Answer from the drawing. Dimensions are ordinates in mm from the lowest x, y and z of the part. A direction names the side the tool comes from. Round coordinates to 2 decimals unless told otherwise and drop trailing zeros. Order: outer loops, then holes, each group sorted by start corner. A loop starts at its lowest first (then second) coordinate and runs counter-clockwise, first axis right, second up. Notation, with made-up numbers: (-6, -23) -> (43, -23) arc R15 cw to (43, -13) -> close; hole circle Ø5 at (-26, -16.5). An arc over 180 degrees is marked (long way). Use a Markdown table: item, result. Add a question column.
Item 1: A cutting plane is placed at B-B, the plane y = 14.5. Determine the outline of the cut face in (x, z).
Item 2: A cutting plane is placed at C-C, the plane y = 5.25. Determine the outline of the cut face in (x, z).
Item 3: Flat-ended cylindrical pins translate along their axes: P1, Ø5, axis at x = 4, z = 2, coming from the +Y side; P2, Ø5, axis at x = 17.5, y = 12, coming from the +Z side; P3, Ø5, axis at x = 8, y = 10, coming from the +Z side; P4, Ø6, axis at y = 15, z = 9.5, coming from the +X side. Find the tip coordinate at first contact, or state that the pin passes through.
Item 4: For a pull along Z with two mould halves and no side action, classify the marked faces 1, 2, 3 and 4 as +Z half, -Z half, draft (parallel to the pull), parting line (faces both ways), or undercut.
Item 5: A cutting plane is placed at D-D, the plane x = 18.5. Determine the outline of the cut face in (y, z).
Item 6: A cutting plane is placed at A-A, the plane x = 2. Determine the outline of the cut face in (y, z).
Item 7: A tool of negligible diameter and unlimited length cuts with its end or side. For the marked faces 5, 6 and 7, from which of +Z, -Z, +X, -X, +Y, -Y can it reach the whole face along a straight path? Write none if from no direction.
Item 8: Find the intervals of material crossed by L1, parallel to X at y = 5.75, z = 11; L2, parallel to Z at x = 11, y = 13.5; L3, parallel to X at y = 7.75, z = 10, in increasing order. Write a range as [from, to].
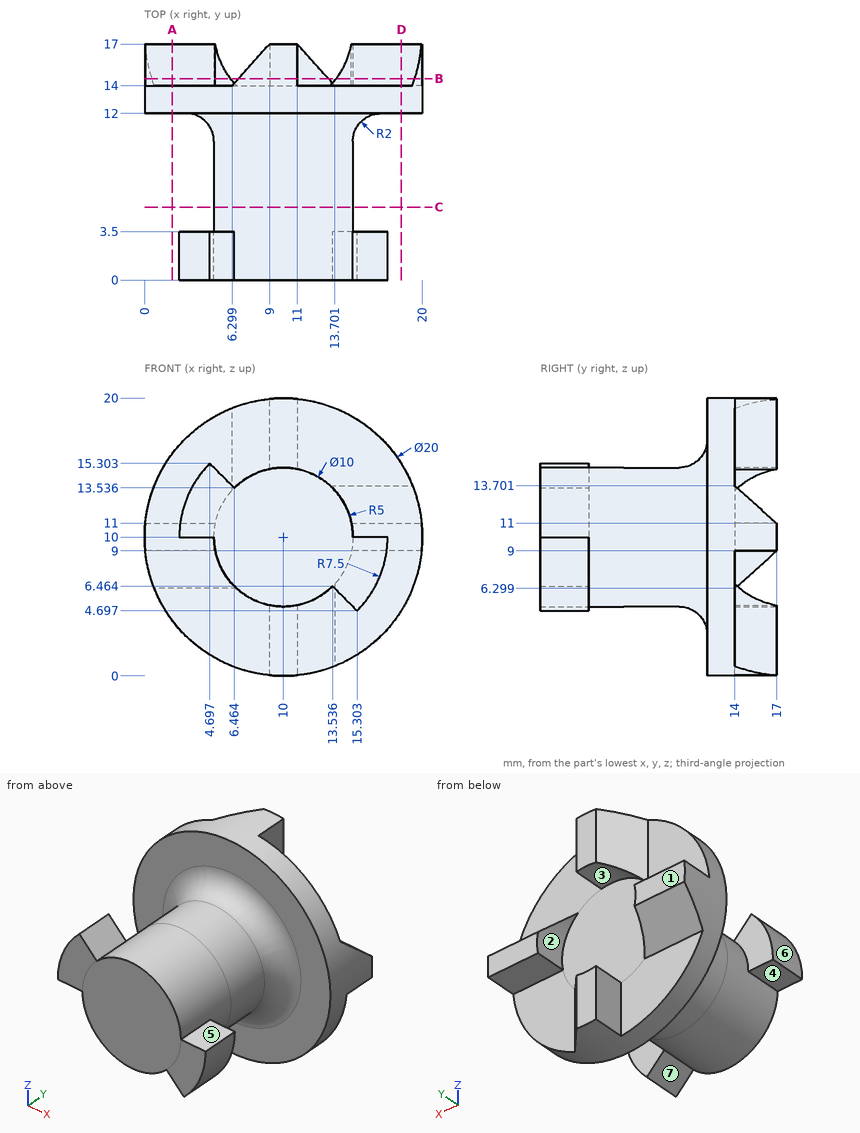
Reported:
| question | item | result |
|---|---|---|
| 1 | outline | (0.05, 11) arc R10 ccw to (0.54, 6.75) -> (6.2, 6.75) arc R5 cw to (5.1, 11) -> close; (6.75, 13.8) arc R5 cw to (11, 14.9) -> (11, 19.95) arc R10 ccw to (6.75, 19.46) -> close; (9, 0.05) arc R10 ccw to (13.25, 0.54) -> (13.25, 6.2) arc R5 cw to (9, 5.1) -> close; (13.8, 13.25) arc R5 cw to (14.9, 9) -> (19.95, 9) arc R10 ccw to (19.46, 13.25) -> close |
| 2 | outline | circle Ø10 at (10, 10) |
| 3 | P1 | y = 14 |
| 3 | P2 | z = 18.66 |
| 3 | P3 | z = 19.99 |
| 3 | P4 | x = 20 |
| 4 | face 1 | draft |
| 4 | face 2 | undercut |
| 4 | face 3 | undercut |
| 4 | face 4 | -Z half |
| 5 | outline | (12, 4.73) -> (14, 4.73) -> (14, 9) -> (17, 9) -> (17, 11) -> (14, 13.7) -> (14, 15.27) -> (12, 15.27) -> close |
| 6 | outline | (12, 4) -> (14, 4) -> (14, 6.3) -> (17, 9) -> (17, 11) -> (14, 11) -> (14, 16) -> (12, 16) -> close |
| 7 | face 5 | +Z, +X, -Y |
| 7 | face 6 | +Z, -X, -Y |
| 7 | face 7 | -Z, -Y |
| 8 | L1 | [5.1, 14.9] |
| 8 | L2 | [0.05, 19.95] |
| 8 | L3 | [5, 15] |
